Geometry: final body of the model. Coordinates: model frame, mm. A direction names the side the tool comes from. Give positions to 0.01 mm unless a question says otherwise; leave off trailing zeros. Loops run counter-clockwise (first coordinate to the right, second up) from the corner with the lowest first, then second, coordinate; pieces in that order, holes last.
```python
from build123d import *

# Parameters (mm, degrees)
SKETCH1_R           = 1.5
BOSS_EXTRUDE1_DEPTH = 4
FILLET1_R           = 3


with BuildPart() as part:
    # Sketch1 → Boss-Extrude1 (new body)
    with BuildSketch(Plane.XY):
        with BuildLine():
            Line((0, 0), (30, 0))
            Line((30, 0), (38, 0))
            Line((38, 0), (38, -8))
            Line((38, -8), (28.91366459, -8))
            ThreePointArc((28.91366459, -8), (18.165902125, -23.874672773), (0, -30))
            Line((0, -30), (0, 0))
        make_face()
        with Locations((4, -26)):
            Circle(SKETCH1_R, mode=Mode.SUBTRACT)
        with Locations((3, -3)):
            Circle(SKETCH1_R, mode=Mode.SUBTRACT)
        with BuildLine():
            ThreePointArc((4.950906496, -17.825221594), (3.907043109, -19.671934682), (5.753756198, -20.715798069))
            ThreePointArc((5.753756198, -20.715798069), (15.340798069, -15.063529288), (20.817285486, -5.375))
            ThreePointArc((20.817285486, -5.375), (19.739916731, -3.547631245), (17.912547976, -4.625))
            ThreePointArc((17.912547976, -4.625), (13.200221594, -12.961641481), (4.950906496, -17.825221594))
        make_face(mode=Mode.SUBTRACT)
    extrude(amount=BOSS_EXTRUDE1_DEPTH)

    # Fillet1
    fillet1_edges = [part.edges().sort_by_distance(p)[0] for p in [
        (0, 0, 2),
        (38, 0, 2),
        (38, -8, 2),
        (28.91366459, -8, 2),
        (0, -30, 2),
    ]]
    fillet(fillet1_edges, radius=FILLET1_R)


solid = part.part
```
Q1. Mould query, pull axis Y, two halves, no side actions, for faces 4 (the face through (19, 0, 2)), 5 (the face through (19.772, -3.556, 1.972)), 6 (the face through (11, -11, 4)). Classes: +Y half, -Y half, draft (parallel to the pull), parting line (faces both ways), or undercut.
Q2. Section query B-B, the plane x = 8. Return loops of the section in (y, z).
Q3. Section query A-A, the plane y = -26. Return loops of the section in (x, z).
Q4. Material intervals for probe 1 along Y at (x, z) = (3.5, 1.85); probe 2 along X at (y, z) = (-18.75, 1.2); probe 3 along Y at (x, z) = (3, 1.7), sorted ascending.
Q5. Pin query (flat end, axial travel): pin 1 Ø2 at (x, y) = (26, -20) entering from -Z; pin 2 Ø1 at (x, z) = (29, 2) entering from -Y. Return the tip coordinate at first contact, or that it passes through.
Q6. Reachability of faces 1 (the face through (13.295, -12.865, 1.972)), 2 (the face through (0, -15, 2)), 3 (the face through (33, -8, 2)) from +Z, -Z, +X, -X, +Y, -Y: full face, straight path, thin tool, end or side. Return the list, or none.
Q7. Section query D-D, the plane x = 27. Return loops of the section in (y, z), and give its area (3 significant figures).
Q8. Section query C-C, the plane z = 2.85. Return loops of the section in (x, y) (1 decimal), and give its area (3 significant figures).
Resolved:
1. face 4: +Y half
1. face 5: undercut
1. face 6: draft
2. outline: (-28.91, 0) - (-19.96, 0) - (-19.96, 4) - (-28.91, 4) - close; (-16.68, 0) - (0, 0) - (0, 4) - (-16.68, 4) - close
3. outline: (0, 0) - (2.5, 0) - (2.5, 4) - (0, 4) - close; (5.5, 0) - (14.97, 0) - (14.97, 4) - (5.5, 4) - close
4. probe 1: y = -29.8 to -27.41, -24.59 to -4.41, -1.59 to 0
4. probe 2: x = 0 to 3.95, 10.52 to 23.42
4. probe 3: y = -29.83 to -27.12, -24.88 to -4.5, -1.5 to 0
5. pin 1: passes through
5. pin 2: stops at y = -9.53
6. face 1: +Z, -Z
6. face 2: +Z, -Z, -X, +Y, -Y
6. face 3: +Z, -Z, +X, -Y
7. outline: (-13.08, 0) - (0, 0) - (0, 4) - (-13.08, 4) - close
7. area: 52.3 mm2
8. outline: (0, -26.8) arc R3 ccw to (3.3, -29.8) arc R30 ccw to (28.3, -10) arc R3 cw to (31.1, -8) - (35, -8) arc R3 ccw to (38, -5) - (38, -3) arc R3 ccw to (35, 0) - (3, 0) arc R3 ccw to (0, -3) - close; hole circle Ø3 at (3, -3); hole circle Ø3 at (4, -26); hole (5, -17.8) arc R1.5 ccw to (5.8, -20.7) arc R21.5 ccw to (20.8, -5.4) arc R1.5 ccw to (17.9, -4.6) arc R18.5 cw to start
8. area: 682 mm2
